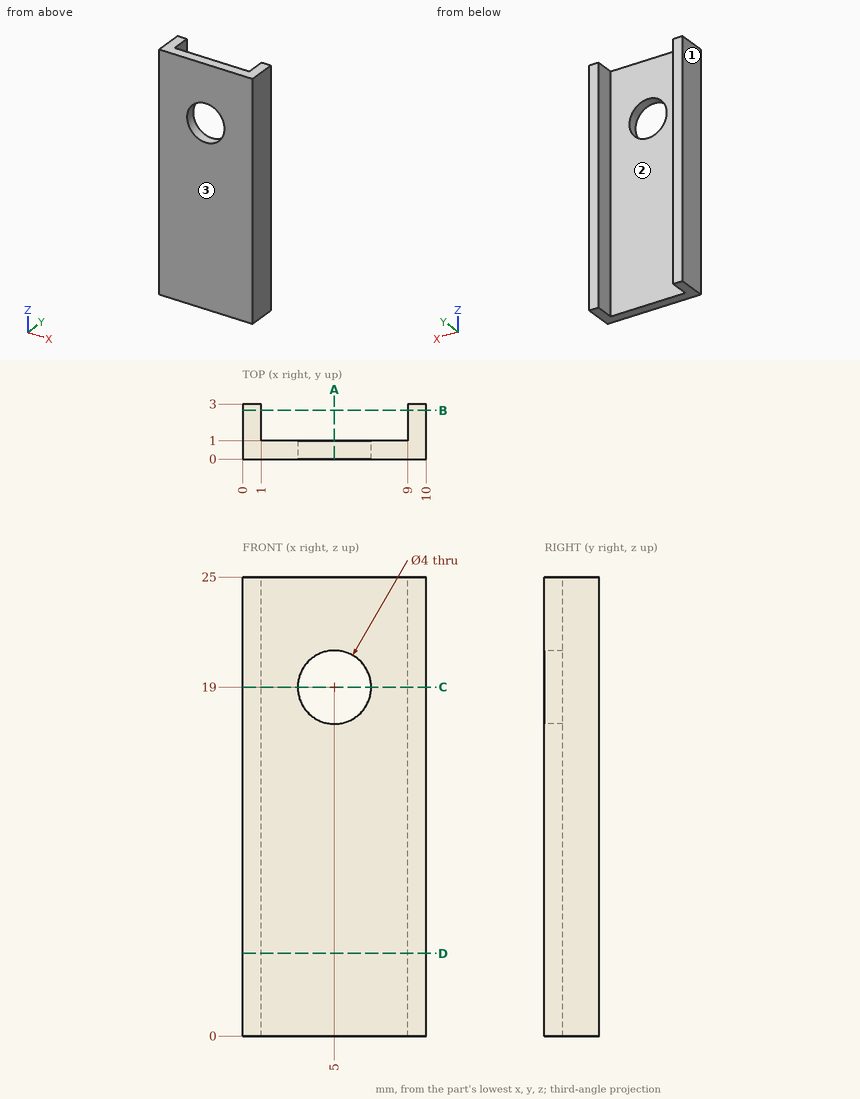
Design review of the part shown in the three views and the two pictorial views. Dimensions are in mm from the part's minimum x, y and z. Round coordinates to 2 decimals unless told otherwise and drop trailing zeros. Order: outer loops, then holes, each group sorted by start corner. A loop starts at its lowest first (then second) coordinate and runs counter-clockwise, first axis right, second up.
(1) Take a section at C-C, the plane z = 19. State the section outline as (x, y) points, plus the area to 3 significant figures.
Working result:
outline: (0, 0) - (3, 0) - (3, 1) - (1, 1) - (1, 3) - (0, 3) - close; (7, 0) - (10, 0) - (10, 3) - (9, 3) - (9, 1) - (7, 1) - close
area: 10.0 mm2
(2) Take a section at D-D, the plane z = 4.5. State the section outline as (x, y) points.
Working result:
outline: (0, 0) - (10, 0) - (10, 3) - (9, 3) - (9, 1) - (1, 1) - (1, 3) - (0, 3) - close
(3) For P1, Ø1.5, axis at x = 5.5, z = 20, coming from the +Y side, flat-tipped, find the tip position at first contact; note if it passes through.
Working result:
P1: passes through
(4) Take a section at A-A, the plane x = 5. State the section outline as (y, z) points.
Working result:
outline: (0, 0) - (1, 0) - (1, 17) - (0, 17) - close; (0, 21) - (1, 21) - (1, 25) - (0, 25) - close
(5) Mouldability with a two-part tool opening along X and no side actions: class the marked faces 1, 2 and 3 as released by +X, released by -X, zero draft, split by the parting line, or undercut.
Working result:
face 1: released by -X
face 2: undercut
face 3: zero draft
(6) Take a section at B-B, the plane y = 2.65. State the section outline as (x, z) points.
Working result:
outline: (0, 0) - (1, 0) - (1, 25) - (0, 25) - close; (9, 0) - (10, 0) - (10, 25) - (9, 25) - close
(7) Wall thickness on L1, parallel to X at y = 2.4, z = 7.75; L2, parallel to Z at x = 5, y = 0.3; L3, parallel to Y at x = 8.75, z = 19.25: over which ranges is each line inside the solid? List them lowest first.
Working result:
L1: x = 0 to 1, 9 to 10
L2: z = 0 to 17, 21 to 25
L3: y = 0 to 1
